```python
from build123d import *

# Parameters (mm, degrees)
SKETCH_1_W      = 25
SKETCH_1_H      = 23
EXTRUDE_1_DEPTH = 1.6
SKETCH_2_R      = 1.25
SKETCH_2_W      = 15
SKETCH_2_H      = 15
EXTRUDE_2_DEPTH = 2
EXTRUDE_3_DEPTH = 2


with BuildPart() as part:
    # Эскиз1 → Бобышка-Вытянуть1 (new body)
    with BuildSketch(Plane.XY):
        with Locations((12.5, 11.5)):
            Rectangle(SKETCH_1_W, SKETCH_1_H)
    extrude(amount=EXTRUDE_1_DEPTH)

    # Эскиз2 → Бобышка-Вытянуть2 (add)
    with BuildSketch(Plane.XY.offset(1.6)):
        with Locations((3.5, 19.5)):
            Circle(SKETCH_2_R)
        with Locations((12.5, 9.5)):
            Rectangle(SKETCH_2_W, SKETCH_2_H)
    extrude(amount=EXTRUDE_2_DEPTH)

    # Эскиз3 → Бобышка-Вытянуть3 (add)
    with BuildSketch(Plane(origin=(0, 0, 0), x_dir=(-1, 0, 0), z_dir=(0, 0, -1))):
        Polygon((-15.5, 23), (-7.5, 23), (-7.5, 7), (-17.5, 7), (-17.5, 21), align=None)
    extrude(amount=EXTRUDE_3_DEPTH)


solid = part.part
```
Here's how the part is built. I have some questions about the finished solid (model axes, mm). A direction names the side the tool comes from. Coordinates: 2 decimals unless noted, no trailing zeros. Write each loop counter-clockwise with the first axis right and the second up, starting at its lowest first coordinate (ties: lowest second). Pieces come first, ordered by that corner, then holes. Notation, with made-up numbers: (79.25, 74) -> (99.25, 74) arc R13 ccw to (99.25, 97) -> close; hole circle Ø5 at (49, 25). An arc over 180 degrees is marked (long way). Use a Markdown table: item, result. Add a question column.
(1) For faces 1 (the flat face through (17.5, 14, -1)), 2 (the flat face through (16.5, 22, -1)), 3 (the cylindrical face through (3.23, 18.28, 2.59)), which set-ups out of +Z, -Z, +X, -X, +Y, -Y let a thin tool reach every point of the face, with its end or its side?
(2) If we section it at D-D, the plane z = -1.45: Write out the boundary of the cut face in (x, y).
(3) Please list where these lines run through material, in increasing order: line 1 (X direction, y = 8.25, z = -1.45); line 2 (Y direction, x = 10.25, z = 2.15); line 3 (Z direction, x = 22.5, y = 7.5).
(4) If we section it at A-A, the plane x = 16: Write out the boundary of the cut face in (y, z), and give its area (3 significant figures).
(5) I'm going to push flat-ended pins straight in: P1, Ø1, axis at x = 13, z = -1, coming from the -Y side; P2, Ø1.5, axis at x = 10, z = 3, coming from the +Y side; P3, Ø1.5, axis at y = 10, z = 2.5, coming from the +X side. Where does each tip first touch, or does it pass through?
(6) If we section it at C-C, the plane y = 4.75: Write out the boundary of the cut face in (x, z), and give its area (3 significant figures).
(7) If we section it at B-B, the plane z = 3: Write out the boundary of the cut face in (x, y).
Outcome:
| question | item | result |
|---|---|---|
| 1 | face 1 | -Z, +X, +Y, -Y |
| 1 | face 2 | -Z, +X, +Y |
| 1 | face 3 | +Z |
| 2 | outline | (7.5, 7) -> (17.5, 7) -> (17.5, 21) -> (15.5, 23) -> (7.5, 23) -> close |
| 3 | line 1 | x = 7.5 to 17.5 |
| 3 | line 2 | y = 2 to 17 |
| 3 | line 3 | z = 0 to 1.6 |
| 4 | outline | (0, 0) -> (7, 0) -> (7, -2) -> (22.5, -2) -> (22.5, 0) -> (23, 0) -> (23, 1.6) -> (17, 1.6) -> (17, 3.6) -> (2, 3.6) -> (2, 1.6) -> (0, 1.6) -> close |
| 4 | area | 97.8 mm^2 |
| 5 | P1 | stops at y = 7 |
| 5 | P2 | stops at y = 17 |
| 5 | P3 | stops at x = 20 |
| 6 | outline | (0, 0) -> (25, 0) -> (25, 1.6) -> (20, 1.6) -> (20, 3.6) -> (5, 3.6) -> (5, 1.6) -> (0, 1.6) -> close |
| 6 | area | 70.0 mm^2 |
| 7 | outline | circle Ø2.5 at (3.5, 19.5); (5, 2) -> (20, 2) -> (20, 17) -> (5, 17) -> close |
